Build history of the part. All positions in model axes, mm. A direction names the side the tool comes from. Give positions to 0.01 mm unless a question says otherwise; leave off trailing zeros. Loops run counter-clockwise (first coordinate to the right, second up) from the corner with the lowest first, then second, coordinate; pieces in that order, holes last.
1) Band-saw the part on B-B on z = -50.8. List the corners of the cut face in (x, y) (3 decimals).
2) Band-saw the part on D-D on x = 18. List the corners of the cut face in (y, z).
3) Wall check: line 1 (X direction, y = 1.35, z = -50.8) (3 decimals); line 2 (X direction, y = 2.3, z = -38.5); line 3 (Z direction, x = -4.5, y = 0.45). Give the ranges that are in metal, low to high.
4) 3-axis set-ups, long thin cutter, end or side, ignore diameter. For faces 5 (the flat face through (-4.762, 1, -36)), 6 (the flat face through (-2, 0, -7)): which of +Z, -Z, +X, -X, +Y, -Y reach the whole face in a straight line?
5) Two-plate mould, pull along X, no slides. Class faces 1 (the cylindrical face through (-23, 1, -20)), 2 (the cylindrical face through (-19.86, 1.25, -19.7)), 3 (the cylindrical face through (0.204, 1.288, -57.147)), 4 (the cylindrical face through (-19.11, 1.25, 16.73)): +X half, -X half, draft (parallel to the pull), parting line (faces both ways), or undercut.
6) Band-saw the part on C-C on y = 1.15. State how many separate pieces and enclosed holes the cut face has, then the cut area to 3 significant figures.
7) Flat gauge pins, fed straight in: P1, Ø10, axis at x = 0, z = 0, coming from the +Y side; P2, Ø1.3, axis at y = 1, z = -40.5, coming from the +X side; P3, Ø0.8, axis at y = 1, z = -30.5, coming from the -X side. Where does each tip first touch, or does it go through?
8) Band-saw the part on A-A on x = 0. List the corners of the cut face in (y, z) (3 decimals).
```python
from build123d import *

# Parameters (mm, degrees)
SKETCH1_R           = 25.4
SKETCH1_R_2         = 6.35
BOSS_EXTRUDE1_DEPTH = 2.54
BOSS_EXTRUDE3_DEPTH = 2.54
CIRPATTERN2_DEPTH   = 2.54
SKETCH4_R           = 3.175
BOSS_EXTRUDE4_DEPTH = 2.54


# Read off the part's stored shape, not the designer's step: CirPattern2
with BuildPart() as part:
    # Sketch1 → Boss-Extrude1 (new body)
    with BuildSketch(Plane(origin=(0, 0, 0), x_dir=(1, 0, 0), z_dir=(0, 1, 0))):
        with Locations(Location((0, 0, 0), (0, 0, 270))):
            Circle(SKETCH1_R)
        with Locations(Location((0, 0, 0), (0, 0, 270))):
            Circle(SKETCH1_R_2, mode=Mode.SUBTRACT)
    extrude(amount=BOSS_EXTRUDE1_DEPTH)

    # Sketch3 → Boss-Extrude3 (add)
    with BuildSketch(Plane(origin=(0, 0, 0), x_dir=(1, 0, 0), z_dir=(0, 1, 0))):
        with BuildLine():
            ThreePointArc((-24.569920792, 6.440418643), (-27.081444643, 7.133180463), (-29.679543147, 6.939388921))
            ThreePointArc((-29.679543147, 6.939388921), (-29.894335347, 5.946353015), (-30.075911618, 4.94671005))
            ThreePointArc((-30.075911618, 4.94671005), (-27.7497424, 3.773420758), (-25.164288447, 3.452330656))
            ThreePointArc((-25.164288447, 3.452330656), (-24.911946122, 4.955294179), (-24.569920792, 6.440418643))
        make_face()
    extrude(amount=BOSS_EXTRUDE3_DEPTH)

    # CirPattern2 outline → CirPattern2 (add)
    with BuildSketch(Plane(origin=(0, 0, 0), x_dir=(1, 0, 0), z_dir=(0, 1, 0))):
        with BuildLine():
            ThreePointArc((-23.413307188, 9.847692448), (-22.780567636, 11.234132732), (-22.06581804, 12.580130138))
            ThreePointArc((-22.06581804, 12.580130138), (-24.312463838, 13.899316875), (-26.872191224, 14.384565994))
            ThreePointArc((-26.872191224, 14.384565994), (-27.336681162, 13.480959278), (-27.77079701, 12.562373718))
            ThreePointArc((-27.77079701, 12.562373718), (-25.8275597, 10.827006393), (-23.413307188, 9.847692448))
        make_face()
        with BuildLine():
            ThreePointArc((-20.066747736, 15.571950275), (-19.096731111, 16.747383705), (-18.057966254, 17.862526553))
            ThreePointArc((-18.057966254, 17.862526553), (-19.886628801, 19.718237812), (-22.233543877, 20.849458666))
            ThreePointArc((-22.233543877, 20.849458666), (-22.916077332, 20.096860444), (-23.573148479, 19.321932378))
            ThreePointArc((-23.573148479, 19.321932378), (-22.145271488, 17.142749435), (-20.066747736, 15.571950275))
        make_face()
        with BuildLine():
            ThreePointArc((-15.571950272, -20.066747733), (-16.747383702, -19.096731108), (-17.86252655, -18.057966251))
            ThreePointArc((-17.86252655, -18.057966251), (-19.718237812, -19.886628801), (-20.849458666, -22.233543877))
            ThreePointArc((-20.849458666, -22.233543877), (-20.096860444, -22.916077332), (-19.321932378, -23.573148479))
            ThreePointArc((-19.321932378, -23.573148479), (-17.142749435, -22.145271488), (-15.571950272, -20.066747733))
        make_face()
        with BuildLine():
            ThreePointArc((-20.235005421, -15.352672585), (-21.119328151, -14.111483918), (-21.927621299, -12.819493908))
            ThreePointArc((-21.927621299, -12.819493908), (-24.193393428, -14.105552875), (-25.893495185, -16.079717258))
            ThreePointArc((-25.893495185, -16.079717258), (-25.343193783, -16.933780702), (-24.764733277, -17.769028835))
            ThreePointArc((-24.764733277, -17.769028835), (-22.290242434, -16.953819621), (-20.235005421, -15.352672585))
        make_face()
        with BuildLine():
            ThreePointArc((-23.51907839, -9.592338172), (-24.052025288, -8.164562418), (-24.498384895, -6.70739424))
            ThreePointArc((-24.498384895, -6.70739424), (-27.019809264, -7.363206831), (-29.172932798, -8.830084481))
            ThreePointArc((-29.172932798, -8.830084481), (-28.862430347, -9.797474903), (-28.519858529, -10.753979241))
            ThreePointArc((-28.519858529, -10.753979241), (-25.918692246, -10.606992964), (-23.51907839, -9.592338172))
        make_face()
        with BuildLine():
            ThreePointArc((-30.464283252, -0.978696039), (-30.41473998, -1.993487379), (-30.331402553, -3.006063733))
            ThreePointArc((-30.331402553, -3.006063733), (-27.780826014, -3.537317266), (-25.200365035, -3.178301765))
            ThreePointArc((-25.200365035, -3.178301765), (-25.34561665, -1.661239483), (-25.399624045, -0.138196738))
            ThreePointArc((-25.399624045, -0.138196738), (-28.00486975, -0.11907041), (-30.464283252, -0.978696039))
        make_face()
    extrude(amount=CIRPATTERN2_DEPTH)

    # Sketch4 → Boss-Extrude4 (add)
    with BuildSketch(Plane(origin=(0, 2.54, 0), x_dir=(1, 0, 0), z_dir=(0, 1, 0))):
        with BuildLine():
            Line((-4.7625, 6.35), (4.7625, 6.35))
            Line((4.7625, 6.35), (4.7625, 46.599869794))
            ThreePointArc((4.7625, 46.599869794), (0, 57.15), (-4.7625, 46.599869794))
            Line((-4.7625, 46.599869794), (-4.7625, 6.35))
        make_face()
        with Locations(Location((0, 50.8, 0), (0, 0, 270))):
            Circle(SKETCH4_R, mode=Mode.SUBTRACT)
    extrude(amount=-BOSS_EXTRUDE4_DEPTH)


solid = part.part
```
Findings below:
1. outline: (-6.35, 0) - (-3.175, 0) - (-3.175, 2.54) - (-6.35, 2.54) - close; (3.175, 0) - (6.35, 0) - (6.35, 2.54) - (3.175, 2.54) - close
2. outline: (0, -17.92) - (2.54, -17.92) - (2.54, 17.92) - (0, 17.92) - close
3. line 1: x = -6.35 to -3.175, 3.175 to 6.35
3. line 2: x = -4.76 to 4.76
3. line 3: z = -55.28 to -4.48, 4.48 to 25
4. face 5: -X, +Y, -Y
4. face 6: +Z, -Z, +X, -X, -Y
5. face 1: -X half
5. face 2: undercut
5. face 3: parting line
5. face 4: undercut
6. separate pieces: 1
6. enclosed holes: 2
6. area: 2,300 mm2
7. P1: passes through
7. P2: stops at x = 4.76
7. P3: stops at x = -4.76
8. outline: (0, -57.15) - (2.54, -57.15) - (2.54, -53.975) - (0, -53.975) - close; (0, -47.625) - (2.54, -47.625) - (2.54, -6.35) - (0, -6.35) - close; (0, 6.35) - (2.54, 6.35) - (2.54, 25.4) - (0, 25.4) - close
